Autodesk Inventor part; units mm, degrees
ref_plane "to_retainer_XY" through (0, 0, -150) normal (0, 0, -1) x (1, 0, 0)
ref_plane "to_retainer_YZ" through (0, 0, -150) normal (1, 0, 0) x (0, -1, 0)
ref_plane "to_retainer_ZX" through (0, 0, -150) normal (0, -1, 0) x (0, 0, -1)
sketch "_____1" plane through (0, 0, 0) normal (0, 0, 1) x (1, 0, 0)
  line L0 (-2.35, 4.9) -> (-2.35, -4.9)
  arc A0 (-2.35, -4.9) -> (-2.15, -5.1) centre (-2.15, -4.9) ccw
  line L1 (-2.15, -5.1) -> (-1.1124, -5.1)
  arc A1 (-1.1124, -5.1) -> (-0.9535, -5.0214) centre (-1.1124, -4.9) ccw
  arc A2 (0.9535, -5.0214) -> (-0.9535, -5.0214) centre (0, -5.75) ccw
  arc A3 (0.9535, -5.0214) -> (1.1124, -5.1) centre (1.1124, -4.9) ccw
  line L2 (1.1124, -5.1) -> (1.2, -5.1)
  arc A4 (1.2, -5.1) -> (1.3, -5) centre (1.2, -5) ccw
  line L3 (1.3, -5) -> (1.3, -4.3536)
  arc A5 (1.3, -4.3536) -> (1.1517, -4.1603) centre (1.1, -4.3536) ccw
  line L4 (1.1517, -4.1603) -> (-0.4083, -3.7433)
  arc A6 (-1.15, -2.7772) -> (-0.4083, -3.7433) centre (-0.15, -2.7772) ccw
  line L5 (-1.15, -2.7772) -> (-1.15, 2.7772)
  arc A7 (-0.4083, 3.7433) -> (-1.15, 2.7772) centre (-0.15, 2.7772) ccw
  line L6 (-0.4083, 3.7433) -> (1.1517, 4.1603)
  arc A8 (1.1517, 4.1603) -> (1.3, 4.3536) centre (1.1, 4.3536) ccw
  line L7 (1.3, 4.3536) -> (1.3, 5)
  arc A9 (1.3, 5) -> (1.2, 5.1) centre (1.2, 5) ccw
  line L8 (1.2, 5.1) -> (1.1124, 5.1)
  arc A10 (1.1124, 5.1) -> (0.9535, 5.0214) centre (1.1124, 4.9) ccw
  arc A11 (-0.9535, 5.0214) -> (0.9535, 5.0214) centre (0, 5.75) ccw
  arc A12 (-0.9535, 5.0214) -> (-1.1124, 5.1) centre (-1.1124, 4.9) ccw
  line L9 (-1.1124, 5.1) -> (-2.15, 5.1)
  arc A13 (-2.15, 5.1) -> (-2.35, 4.9) centre (-2.15, 4.9) ccw
extrude "Extrusion1" add sketch "_____1" against normal blind 150
sketch "_____2" plane through (-2.35, 0, 0) normal (1, 0, 0) x (0, 0, -1)
  line L0 (1.4, 1.5) -> (1.4, -1.5)
  line L1 (1.4, -1.5) -> (5.9, -1.5)
  line L2 (5.9, -1.5) -> (5.9, 1.5)
  line L3 (5.9, 1.5) -> (1.4, 1.5)
extrude "Extrusion2" cut sketch "_____2" along normal blind 1.2
sketch "_____3" plane through (-2.35, 0, 0) normal (1, 0, 0) x (0, 0, -1)
  line L0 (144.1, 1.5) -> (144.1, -1.5)
  line L1 (144.1, -1.5) -> (148.6, -1.5)
  line L2 (148.6, -1.5) -> (148.6, 1.5)
  line L3 (148.6, 1.5) -> (144.1, 1.5)
extrude "Extrusion3" cut sketch "_____3" along normal blind 1.2
sketch "_____4" plane through (0, 0, 0) normal (0, 1, 0) x (1, 0, 0)
  line L0 (-2.35, 1.4) -> (-1.15, 1.4)
  line L1 (-1.15, 1.4) -> (0.65, 4.9)
  line L2 (0.65, 4.9) -> (0.65, 5.9)
  line L3 (0.65, 5.9) -> (-0.55, 5.9)
  line L4 (-0.55, 5.9) -> (-0.55, 4.9)
  line L5 (-0.55, 4.9) -> (-2.35, 1.4)
extrude "Extrusion4" add sketch "_____4" along normal mid plane 3
sketch "_____5" plane through (0, 0, 0) normal (0, 1, 0) x (1, 0, 0)
  line L0 (-2.35, 148.6) -> (-0.55, 145.1)
  line L1 (-0.55, 145.1) -> (-0.55, 144.1)
  line L2 (-0.55, 144.1) -> (0.65, 144.1)
  line L3 (0.65, 144.1) -> (0.65, 145.1)
  line L4 (0.65, 145.1) -> (-1.15, 148.6)
  line L5 (-1.15, 148.6) -> (-2.35, 148.6)
extrude "Extrusion5" add sketch "_____5" along normal mid plane 3
sketch "_____6" plane through (0, 0, 0) normal (0, 1, 0) x (1, 0, 0)
  line L0 (-1.15, 12) -> (-2.35, 12)
  line L1 (-2.35, 12) -> (-2.35, 13.3)
  line L2 (-2.35, 13.3) -> (-2.1065, 13.0565)
  line L3 (-2.1065, 13.0565) -> (-1.3935, 13.0565)
  line L4 (-1.3935, 13.0565) -> (-1.15, 13.3)
  line L5 (-1.15, 13.3) -> (-1.15, 12)
  line L6 (-1.15, 12) -> (-2.35, 12)
revolve "Revolution1" cut sketch "_____6" angle 360 about axis through (-1.15, 0, -12) along (1, 0, 0)
thread "Thread1"
pattern_linear "Rectangular Pattern1" count 2 spacing 126 along (0, 0, -1) of "Revolution1"
sketch "_____10" plane through (0, 0, 0) normal (0, 1, 0) x (1, 0, 0)
  line L0 (-1.15, 75) -> (-2.35, 75)
  line L1 (-2.35, 75) -> (-2.35, 76.3)
  line L2 (-2.35, 76.3) -> (-2.1065, 76.0565)
  line L3 (-2.1065, 76.0565) -> (-1.3935, 76.0565)
  line L4 (-1.3935, 76.0565) -> (-1.15, 76.3)
  line L5 (-1.15, 76.3) -> (-1.15, 75)
  line L6 (-1.15, 75) -> (-2.35, 75)
revolve "Revolution2" cut sketch "_____10" angle 360 about axis through (-1.15, 0, -75) along (1, 0, 0)
thread "Thread2"
sketch "Sketch8" plane through (-1.15, -2.7772, 0) normal (1, 0, 0) x (0, 0, -1)
  point P0 (24, 2.7772)
hole "Hole1" at (-1.15, 0, -24) direction (-1, 0, 0) diameter 2.8 depth 1.2
sketch "_____8" plane through (-1.15, 0, 0) normal (1, 0, 0) x (0, 0, -1)
  arc A0 (121.8, 1.4) -> (121.8, -1.4) centre (121.8, 0) ccw
  line L0 (121.8, -1.4) -> (122.2, -1.4)
  arc A1 (122.2, -1.4) -> (122.2, 1.4) centre (122.2, 0) ccw
  line L1 (122.2, 1.4) -> (121.8, 1.4)
extrude "Extrusion6" cut sketch "_____8" against normal blind 1.2
ref_plane "to_retainer_XY" through (0, 0, -150) normal (0, 0, -1) x (1, 0, 0)
ref_plane "to_retainer_YZ" through (0, 0, -150) normal (1, 0, 0) x (0, -1, 0)
ref_plane "to_retainer_ZX" through (0, 0, -150) normal (0, -1, 0) x (0, 0, -1)
properties part number "SSRC215_ir" material "ステンレス鋼"
The model under review builds one solid part; all positions refer to its coordinate system, in mm. A direction names the side the tool comes from. Round coordinates to 2 decimals unless told otherwise and drop trailing zeros. Write each loop counter-clockwise with the first axis right and the second up, starting at its lowest first coordinate (ties: lowest second). Pieces come first, ordered by that corner, then holes. Notation, with made-up numbers: (31.25, -25.75) - (88.25, -25.75) arc R33 ccw to (88.25, 6.25) - close; hole circle Ø2 at (20.5, -31). An arc over 180 degrees is marked (long way). Answer as CSV lines item,"result". Start each with the question number.
(1) For pin 1 Ø0.9 at (x, z) = (0, -147) entering from -Y; pin 2 Ø1.3 at (x, y) = (0, -0.5) entering from +Z; pin 3 Ø0.5 at (y, z) = (0.5, -144.5) entering from -X, all flat-tipped, find the tip position at first contact; note any pin that passes through.
(2) For faces 1 (the flat face through (-0.26, -0.02, -3.13)), 2 (the flat face through (-1.46, -0.02, -146.87)), 3 (the flat face through (-1.4, 0.1, -150)), 4 (the flat face through (-0.24, -0.02, -146.83)), list the 3-axis set-ups (+Z, -Z, +X, -X, +Y, -Y) from which the entire face can be reached by the end or side of a thin tool; tool diameter is ignored.
(3) To check wall thickness, follow line 1 (Y direction, x = -1.95, z = -75); line 2 (Y direction, x = -1.85, z = -24); line 3 (X direction, y = -4.25, z = -95). State the ranges of each line that lie inside material, in increasing order.
(4) We need section A-A on z = -15. State the section outline as (x, y) points, plus the area to 3 significant figures.
(5) Draft analysis for pull direction Y (two halves, no side actions). For faces 5 (the flat face through (-1.44, -0.02, -3.17)), 6 (the flat face through (-2.35, 1.2, -74)), state which applies: pulls with the +Y half, pulls with the -Y half, needs draft (parallel to the pull), parting line crosses it, or undercut.
Worked answers:
1,pin 1,"y = -4.64"
1,pin 2,"z = -2.37"
1,pin 3,"x = -0.55"
2,face 1,"+Z, +X"
2,face 2,"-X"
2,face 3,"-Z, +X, -X, +Y, -Y"
2,face 4,"-Z, +X"
3,line 1,"-5.1 to -1.06, 1.06 to 5.1"
3,line 2,"-5.1 to -1.4, 1.4 to 5.1"
3,line 3,"-2.35 to 1.27"
4,outline,"(-2.35, -4.9) arc R0.2 ccw to (-2.15, -5.1) - (-1.11, -5.1) arc R0.2 ccw to (-0.95, -5.02) arc R1.2 cw to (0.95, -5.02) arc R0.2 ccw to (1.11, -5.1) - (1.2, -5.1) arc R0.1 ccw to (1.3, -5) - (1.3, -4.35) arc R0.2 ccw to (1.15, -4.16) - (-0.41, -3.74) arc R1 cw to (-1.15, -2.78) - (-1.15, 2.78) arc R1 cw to (-0.41, 3.74) - (1.15, 4.16) arc R0.2 ccw to (1.3, 4.35) - (1.3, 5) arc R0.1 ccw to (1.2, 5.1) - (1.11, 5.1) arc R0.2 ccw to (0.95, 5.02) arc R1.2 cw to (-0.95, 5.02) arc R0.2 ccw to (-1.11, 5.1) - (-2.15, 5.1) arc R0.2 ccw to (-2.35, 4.9) - close"
4,area,"16.9 mm²"
5,face 5,"undercut"
5,face 6,"needs draft"
